Drawing for the job (mm, zero at the part's lowest x, y, z). Coordinates: 2 decimals unless noted, no trailing zeros. Order: outer loops, then holes, each group sorted by start corner. A loop starts at its lowest first (then second) coordinate and runs counter-clockwise, first axis right, second up. Notation, with made-up numbers: (62, 64.5) -> (108, 64.5) arc R29 cw to (108, 93.5) -> close; hole circle Ø7 at (64, 65). An arc over 180 degrees is marked (long way). Write each question's results on one line, items separated by ' | '.
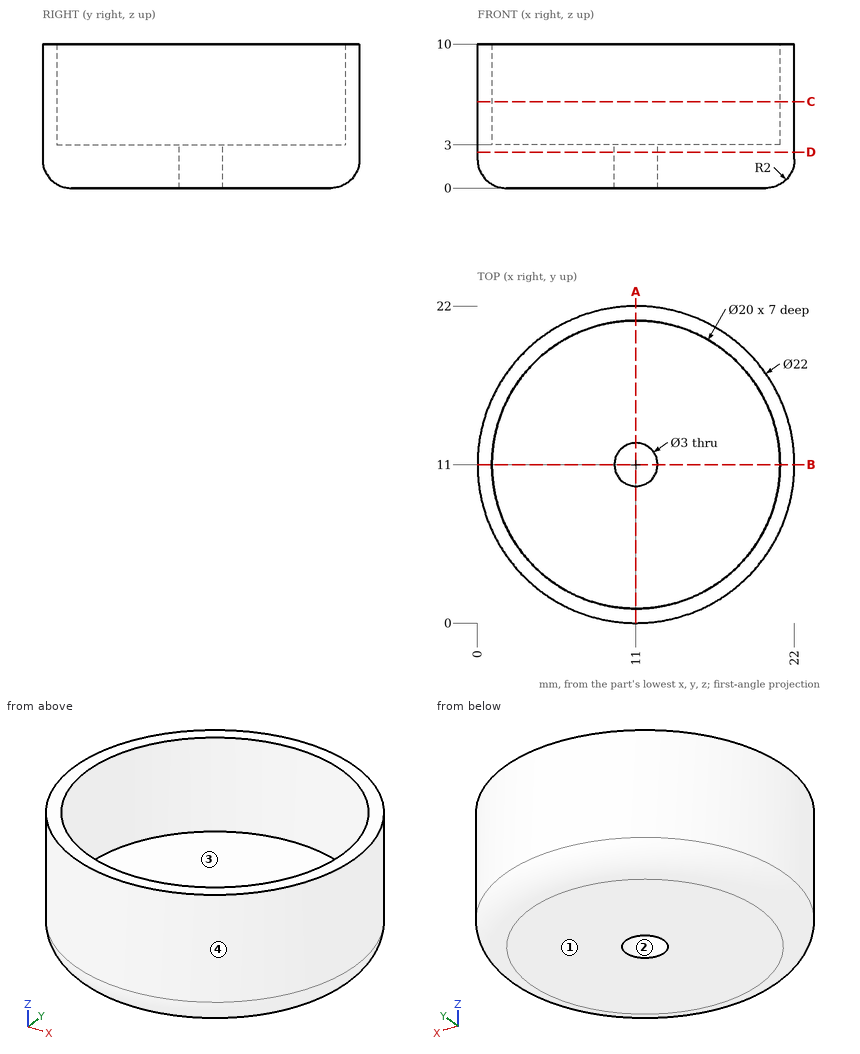
Item 1: Drill centre lines: line 1 (Y direction, x = 11, z = 6.25); line 2 (Y direction, x = 11, z = 2.1); line 3 (Z direction, x = 15, y = 17). Where is each one in solid material? Low to high. Write a range as from..to.
Answer:
line 1: y = 0..1, 21..22 | line 2: y = 0..9.5, 12.5..22 | line 3: z = 0..3
Item 2: Slice it at A-A, the plane x = 11. List the corners of the cut face in (y, z), and give its area (3 significant figures).
Answer:
outline: (0, 2) arc R2 ccw to (2, 0) -> (9.5, 0) -> (9.5, 3) -> (1, 3) -> (1, 10) -> (0, 10) -> close; (12.5, 0) -> (20, 0) arc R2 ccw to (22, 2) -> (22, 10) -> (21, 10) -> (21, 3) -> (12.5, 3) -> close | area: 69.3 mm^2
Item 3: Pull direction Y, two halves, no side cores. Call the marked faces 1, 2, 3 and 4: released by +Y, released by -Y, zero draft, split by the parting line, or undercut.
Answer:
face 1: zero draft | face 2: undercut | face 3: undercut | face 4: split by the parting line
Item 4: Slice it at D-D, the plane z = 2.5. List the corners of the cut face in (x, y), and give its area (3 significant figures).
Answer:
outline: circle Ø22 at (11, 11); hole circle Ø3 at (11, 11) | area: 373 mm^2
Item 5: Pin check, flat tips, straight feed: pin 1 (1 mm diameter, centred on y = 17.5, z = 5.5, fed in from -X); pin 2 (2 mm diameter, centred on y = 7.5, z = 5.5, fed in from +X); pin 3 (4 mm diameter, centred on x = 11, y = 11, fed in from +Z). Stop position of each tip, or through.
Answer:
pin 1: stops at x = 1.78 | pin 2: stops at x = 21.71 | pin 3: stops at z = 3
Item 6: Slice it at C-C, the plane z = 6. List the corners of the cut face in (x, y).
Answer:
outline: circle Ø22 at (11, 11); hole circle Ø20 at (11, 11)
